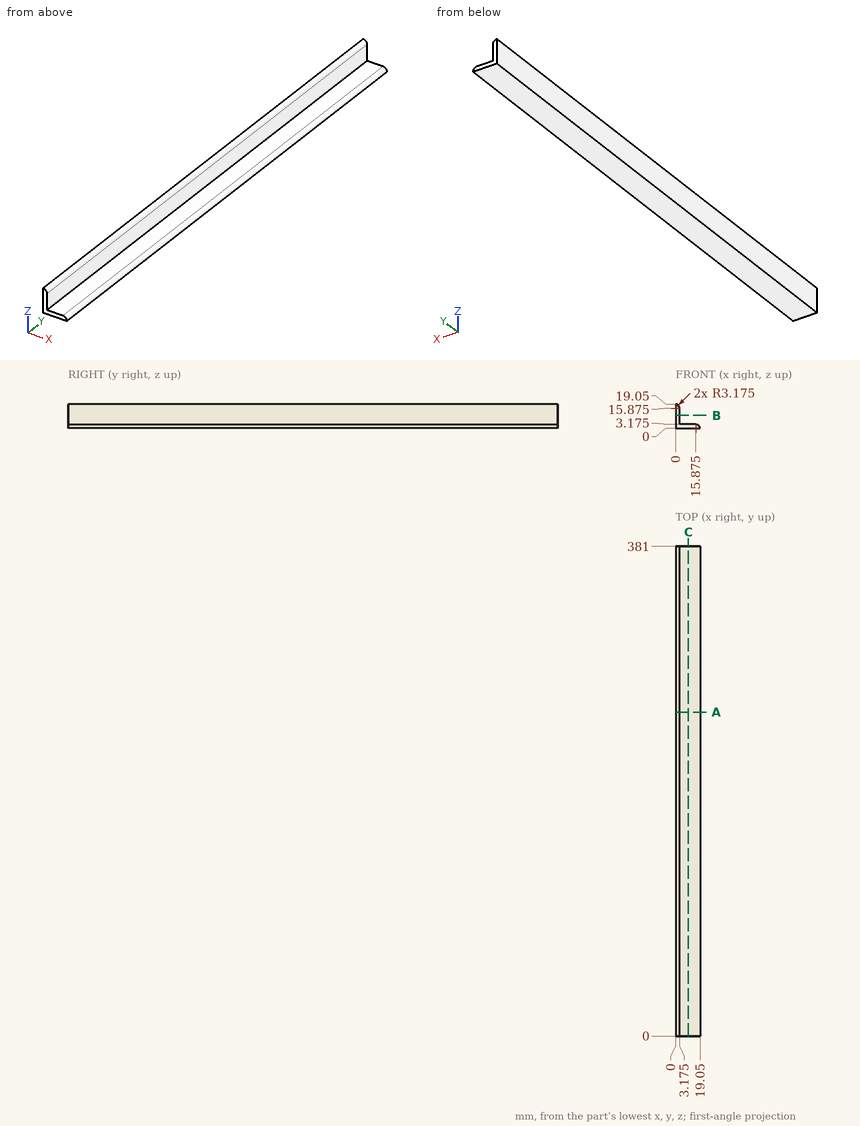
Can you work these out from the drawing? Everything is in mm from the part's minimum corner. Give positions to 0.01 mm unless a question says otherwise; leave off trailing zeros. Order: outer loops, then holes, each group sorted by start corner. A loop starts at its lowest first (then second) coordinate and runs counter-clockwise, first axis right, second up.
Item 1: If we section it at A-A, the plane y = 252: Write out the boundary of the cut face in (x, z) (3 decimals).
Item 2: If we section it at C-C, the plane x = 10: Write out the boundary of the cut face in (y, z) (3 decimals).
Item 3: I'm going to push flat-ended pins straight in: pin 1 (3 mm diameter, centred on y = 272, z = 17, fed in from +X) (3 decimals); pin 2 (4 mm diameter, centred on x = 6.5, y = 192.5, fed in from -Z); pin 3 (4 mm diameter, centred on x = 4.5, y = 130.5, fed in from +Z); pin 4 (10 mm diameter, centred on x = 6.5, y = 253.5, fed in from +Z). Where does each tip first touch, or does it pass through?
Item 4: If we section it at B-B, the plane z = 10.25: Write out the boundary of the cut face in (x, y) (3 decimals), plus the area to 3 significant figures.
Item 5: I need wall thicknesses on line 1 (X direction, y = 324, z = 9.75) (3 decimals); line 2 (Z direction, x = 2.5, y = 143). Which ranges of each line are inside material? Lowest first, please.
Values:
1. outline: (0, 0) - (19.05, 0) arc R3.175 ccw to (15.875, 3.175) - (3.175, 3.175) - (3.175, 15.875) arc R3.175 ccw to (0, 19.05) - close
2. outline: (0, 0) - (381, 0) - (381, 3.175) - (0, 3.175) - close
3. pin 1: stops at x = 3.175
3. pin 2: stops at z = 0
3. pin 3: stops at z = 17.83
3. pin 4: stops at z = 18.67
4. outline: (0, 0) - (3.175, 0) - (3.175, 381) - (0, 381) - close
4. area: 1,210 mm2
5. line 1: x = 0 to 3.175
5. line 2: z = 0 to 17.83
